Build history of the part. All positions in model axes, mm. A direction names the side the tool comes from. Give positions to 0.01 mm unless a question says otherwise; leave off trailing zeros. Order: outer loops, then holes, each group sorted by start corner. A loop starts at its lowest first (then second) coordinate and runs counter-clockwise, first axis right, second up. Notation, with made-up numbers: M 80,-23.5 L 126,-23.5 A26 ccw 126,-8.5 Z; hole C -9,-20 d2. An arc over 180 degrees is marked long. One line per item, written item: value.
from build123d import *

# Parameters (mm, degrees)
EXTRUDE_1_DEPTH     = 250
SKETCH_2_R          = 1.75
SKETCH_2_R_2        = 1.6
CUT_EXTRUDE_1_DEPTH = 252.352407907
SKETCH_3_R          = 3.25
CUT_EXTRUDE_2_DEPTH = 3


with BuildPart() as part:
    # 草图1 → 凸台-拉伸1 (new body)
    with BuildSketch(Plane.XY):
        with BuildLine():
            Line((-6.044750958, 8.167376983), (0, 8.167376983))
            Line((0, 8.167376983), (0, 6.376329748))
            ThreePointArc((0, 6.376329748), (2, 4.376329748), (0, 2.376329748))
            Line((0, 2.376329748), (0, -1.232623017))
            Line((0, -1.232623017), (15.910498084, -1.232623017))
            Line((15.910498084, -1.232623017), (15.910498084, 2.376329748))
            ThreePointArc((15.910498084, 2.376329748), (13.910498084, 4.376329748), (15.910498084, 6.376329748))
            Line((15.910498084, 6.376329748), (15.910498084, 8.167376983))
            Line((15.910498084, 8.167376983), (21.955249042, 8.167376983))
            Line((21.955249042, 8.167376983), (21.955249042, -5.832623017))
            Line((21.955249042, -5.832623017), (-6.044750958, -5.832623017))
            Line((-6.044750958, -5.832623017), (-6.044750958, 8.167376983))
        make_face()
    extrude(amount=EXTRUDE_1_DEPTH)

    # 草图2 → 切除-拉伸1 (cut, through all)
    with BuildSketch(Plane.XZ.offset(5.832623017)):
        with Locations((7.955249042, 215)):
            Circle(SKETCH_2_R)
        with Locations((7.955249042, 155)):
            Circle(SKETCH_2_R)
        with Locations((7.955249042, 95)):
            Circle(SKETCH_2_R)
        with Locations((7.955249042, 35)):
            Circle(SKETCH_2_R)
        with Locations((7.955249042, -25)):
            Circle(SKETCH_2_R)
        with Locations((7.955249042, -85)):
            Circle(SKETCH_2_R)
        with Locations((7.955249042, 10)):
            Circle(SKETCH_2_R_2)
        with Locations((7.955249042, 240)):
            Circle(SKETCH_2_R_2)
    extrude(amount=-CUT_EXTRUDE_1_DEPTH, mode=Mode.SUBTRACT)

    # 草图3 → 切除-拉伸2 (cut)
    with BuildSketch(Plane(origin=(0, -1.232623017, 0), x_dir=(1, 0, 0), z_dir=(0, 1, 0))):
        with Locations(Location((7.955249042, -35, 0), (0, 0, 270))):
            Circle(SKETCH_3_R)
        with Locations(Location((7.955249042, -95, 0), (0, 0, 270))):
            Circle(SKETCH_3_R)
        with Locations(Location((7.955249042, -155, 0), (0, 0, 270))):
            Circle(SKETCH_3_R)
        with Locations(Location((7.955249042, -215, 0), (0, 0, 270))):
            Circle(SKETCH_3_R)
        with Locations((7.955249042, -275)):
            Circle(SKETCH_3_R)
        with Locations(Location((7.955249042, -240, 0), (0, 0, 270))):
            Circle(SKETCH_3_R)
        with Locations(Location((7.955249042, -10, 0), (0, 0, 270))):
            Circle(SKETCH_3_R)
    extrude(amount=-CUT_EXTRUDE_2_DEPTH, mode=Mode.SUBTRACT)


solid = part.part
1) Drill centre lines: probe 1 along X at (y, z) = (-3.15, 35); probe 2 along X at (y, z) = (4, 153); probe 3 along Y at (x, z) = (15.75, 168). Where is each one in solid material? Low to high. Write a range as from..to.
Check values:
probe 1: -6.04..4.71, 11.21..21.96
probe 2: -6.04..1.96, 13.95..21.96
probe 3: -5.83..-1.23, 2.38..6.37
2) Pin check, flat tips, straight feed: pin 1 (5 mm diameter, centred on x = 8, z = 240.5, fed in from +Y); pin 2 (8.5 mm diameter, centred on x = 7.96, z = 155, fed in from +Y). Stop position of each tip, or through.
Check values:
pin 1: y = -4.23
pin 2: y = -1.23
3) Mould opens along Z. For faces 1 (the face through (8, -2, 0)), 2 (the face through (21.955, 1, 123)), 3 (the face through (6.6, -4.233, 11.4)) say: released by +Z, released by -Z, zero draft, split by the parting line, or undercut.
Check values:
face 1: released by -Z
face 2: zero draft
face 3: undercut
4) Saw through at A-A, the plane z = 202.5. Write the cut outline in (x, y), then the cut area to 3 significant figures.
Check values:
outline: M -6.04,-5.83 L 21.96,-5.83 L 21.96,8.17 L 15.91,8.17 L 15.91,6.38 A2 ccw 15.91,2.38 L 15.91,-1.23 L 0,-1.23 L 0,2.38 A2 ccw 0,6.38 L 0,8.17 L -6.04,8.17 Z
area: 255 mm^2
5) Tool access for faces 4 (the face through (8, -5.833, 123)), 5 (the face through (2, 4.4, 123.2)), 6 (the face through (8.93, -2.71, 158.1)): list every direction of +Z, -Z, +X, -X, +Y, -Y with a clear straight run to the whole face (end or side of a thin tool).
Check values:
face 4: +Z, -Z, +X, -X, -Y
face 5: +Z, -Z
face 6: +Y
